Input: part model. Units: mm. Frame: model coordinates. A direction names the side the tool comes from. Give positions to 0.01 mm unless a question says otherwise; leave off trailing zeros. Write each loop counter-clockwise with the first axis right and the second up, starting at its lowest first coordinate (ties: lowest second). Pieces come first, ordered by that corner, then holes. Notation, with made-up numbers: (23.5, 30.25) -> (68.5, 30.25) arc R24 ccw to (68.5, 65.25) -> close; hole circle Ø2 at (67.5, 47.5). An arc over 180 degrees is marked (long way). Return JSON: item names as keys, results as strings. Group by question number.
Item 1: Line query: line 1 (Z direction, x = -66, y = -6); line 2 (X direction, y = -4.5, z = -11); line 3 (X direction, y = -10.5, z = -43.5). Output: solid intervals per line, ascending. Write a range as [from, to].
Item 2: Pin query (flat end, axial travel): P1, Ø4, axis at y = -3.5, z = -18.5, coming from the +X side; P2, Ø3, axis at y = -4, z = -30.5, coming from the -X side; P3, Ø4, axis at y = -11, z = -18.5, coming from the -X side. Return the tip coordinate at first contact, or that it passes through.
Item 3: Section A-A, the plane x = -45.5. Return loops of the section in (y, z).
Item 4: Section B-B, the plane x = -37.5. Return loops of the section in (y, z), then the cut area to 3 significant figures.
Item 5: Mould query, pull axis Y, two halves, no side actions, for faces 1 (the face through (-22.23, -12.48, -28.24)), 2 (the face through (-40.222, -8.326, 7.827)), 3 (the face through (-27.41, -6.27, 5.53)). Classes: released by +Y, released by -Y, zero draft, split by the parting line, or undercut.
Item 6: Set-up query: faces 4 (the face through (-54, -6, 6.797)), 5 (the face through (-20.79, -0.22, -26.89)), 6 (the face through (-46, -9.05, 8)). Return all of +Z, -Z, +X, -X, +Y, -Y with unobstructed straight access to the full face (end or side cutting, diameter ignored); none if empty.
Item 7: Section C-C, the plane y = -2.75. Return loops of the section in (x, z).
from build123d import *

# Parameters (mm, degrees)
F1_DEPTH = 12.7
F3_DEPTH = 25.4
F4_R     = 0.762


with BuildPart() as f1:
    # F0 (on Front) → F1 (new body)
    with BuildSketch(Plane.XZ):
        with BuildLine():
            Line((-30.084311, 8.829161), (-69.908474, 8.829161))
            Line((-69.908474, 8.829161), (-69.879254, 6.797161))
            Line((-69.879254, 6.797161), (-30.769229, 6.797161))
            ThreePointArc((-30.769229, 6.797161), (-27.373303, 5.495266), (-25.717982, 2.256878))
            Line((-25.717982, 2.256878), (-19.204397, -58.704096))
            Line((-19.204397, -58.704096), (-17.183898, -58.488209))
            Line((-17.183898, -58.488209), (-23.770251, 3.153808))
            ThreePointArc((-23.770251, 3.153808), (-25.839402, 7.201793), (-30.084311, 8.829161))
        make_face()
    extrude(amount=F1_DEPTH)

    # F2 (on face) → F3 (cut)
    with BuildSketch(Plane.XY.offset(8.829161)):
        with BuildLine():
            Line((-41.998038, -3.787424), (-50.117151, -3.787424))
            ThreePointArc((-50.117151, -3.787424), (-51.913202, -4.531373), (-52.657151, -6.327424))
            Line((-52.657151, -6.327424), (-52.657151, -6.510304))
            ThreePointArc((-52.657151, -6.510304), (-51.913202, -8.306355), (-50.117151, -9.050304))
            Line((-50.117151, -9.050304), (-41.998038, -9.050304))
            ThreePointArc((-41.998038, -9.050304), (-40.201987, -8.306355), (-39.458038, -6.510304))
            Line((-39.458038, -6.510304), (-39.458038, -6.327424))
            ThreePointArc((-39.458038, -6.327424), (-40.201987, -4.531373), (-41.998038, -3.787424))
        make_face()
    extrude(amount=-F3_DEPTH, mode=Mode.SUBTRACT)

    # F4
    f4_edges = [f1.edges().sort_by_distance(p)[0] for p in [
        (-49.996392, -12.7, 8.829161),
        (-17.183898, -6.35, -58.488209),
        (-50.324242, -12.7, 6.797161),
        (-20.477074, 0, -27.6672),
        (-22.461189, 0, -28.223609),
        (-18.194148, 0, -58.596152),
        (-19.204397, -6.35, -58.704096),
        (-18.194148, -12.7, -58.596152),
        (-69.879254, -6.35, 6.797161),
        (-69.893864, -12.7, 7.813161),
        (-69.908474, -6.35, 8.829161),
        (-69.893864, 0, 7.813161),
        (-25.839402, 0, 7.201793),
        (-25.839402, -12.7, 7.201793),
    ]]
    fillet(f4_edges, radius=F4_R)


solid = f1.part
Answer below:
{
 "1": {"line 1": "z = [6.8, 8.83]", "line 2": "x = [-24.3, -22.26]", "line 3": "x = [-20.83, -18.79]"},
 "2": {"P1": "stops at x = -21.24", "P2": "stops at x = -22.38", "P3": "stops at x = -23.71"},
 "3": {"outline": "(-12.7, 7.56) arc R0.76 ccw to (-11.94, 6.8) -> (-9.05, 6.8) -> (-9.05, 8.83) -> (-11.94, 8.83) arc R0.76 ccw to (-12.7, 8.07) -> close; (-3.79, 6.8) -> (-0.76, 6.8) arc R0.76 ccw to (0, 7.56) -> (0, 8.07) arc R0.76 ccw to (-0.76, 8.83) -> (-3.79, 8.83) -> close"},
 "4": {"outline": "(-12.7, 7.56) arc R0.76 ccw to (-11.94, 6.8) -> (-0.76, 6.8) arc R0.76 ccw to (0, 7.56) -> (0, 8.07) arc R0.76 ccw to (-0.76, 8.83) -> (-11.94, 8.83) arc R0.76 ccw to (-12.7, 8.07) -> close", "area": "25.3 mm2"},
 "5": {"face 1": "released by -Y", "face 2": "undercut", "face 3": "zero draft"},
 "6": {"face 4": "-Z, -X, +Y, -Y", "face 5": "+Z, +X, +Y", "face 6": "+Z, -Z"},
 "7": {"outline": "(-69.9, 8.06) -> (-69.89, 7.55) arc R0.76 ccw to (-69.13, 6.8) -> (-30.77, 6.8) arc R5.08 cw to (-25.72, 2.26) -> (-19.29, -57.95) arc R0.76 ccw to (-18.45, -58.62) -> (-17.94, -58.57) arc R0.76 ccw to (-17.26, -57.73) -> (-23.77, 3.15) arc R6.35 ccw to (-30.08, 8.83) -> (-69.14, 8.83) arc R0.76 ccw to start"}
}
